Geometry check sheet. Reference: the model listing, model coordinates, mm. A direction names the side the tool comes from. Give positions to 0.01 mm unless a question says otherwise; leave off trailing zeros. Loops run counter-clockwise (first coordinate to the right, second up) from the corner with the lowest first, then second, coordinate; pieces in that order, holes last. Notation, with made-up numbers: (88, 71) - (111, 71) arc R15 ccw to (111, 97) - close; hole circle Ø2 at (29, 3.25). An arc over 180 degrees is marked (long way). Use a Markdown table: item, result. Add a question column.
1. Depth check by flat-ended pin: P1, Ø1.5, axis at y = -0.5, z = -3.5, coming from the +X side; P2, Ø1.5, axis at y = 0, z = -12.5, coming from the -X side; P3, Ø0.9, axis at x = 53.5, y = 0, coming from the -Z side. Enter the tip coordinate at first touch or a pass-through.
2. Cross-section at D-D on x = -9.45. Enter the section's corners in (y, z), and give its area (3 significant figures).
3. Set-up check for faces 1 (the flat face through (15, 0, -24)), 2 (the flat face through (0, 0, 7.9)), 3 (the flat face through (11.6, 0, -6)): record each of +Z, -Z, +X, -X, +Y, -Y from which the full face is reachable in a straight line by a thin tool's end or side.
4. Draft check along X on faces 4 (the flat face through (-43.4, 0, -6)), 5 (the flat face through (45, 0, 9)), 6 (the flat face through (52, 0, -22.6)). Enter one of: pulls with the +X half, pulls with the -X half, needs draft (parallel to the pull), parting line crosses it, or undercut.
5. Cross-section at B-B on y = 0.6. Count the separate pieces of the cut face and the enclosed holes in it, and give its area (3 significant figures).
6. Cross-section at A-A on x = -24.45. Enter the section's corners in (y, z), and give its area (3 significant figures).
7. Material ranges on L1, parallel to X at y = 0.8, z = -23.5; L2, parallel to Z at x = -48, y = -0.3; L3, parallel to Z at x = -14, y = 0.8, recorded low to high.
from build123d import *

# Parameters (mm, degrees)
EXTRUDE_1_DEPTH        = 1.5
SKETCH_2_W             = 94.999999969
SKETCH_2_H             = 7.3
CUT_EXTRUDE_1_DEPTH    = 10
SKETCH_4_W             = 94.999999969
SKETCH_4_H             = 4
CUT_EXTRUDE_3_DEPTH    = 10
SKETCH_5_W             = 30
SKETCH_5_H             = 3
EXTRUDE_2_DEPTH        = 3
EXTRUDE_3_DEPTH        = 3
SKETCH_7_R             = 1
CUT_EXTRUDE_4_DEPTH    = 3
CUT_EXTRUDE_5_DEPTH    = 5
PATTERN_LINEAR_1_COUNT = 19
PATTERN_LINEAR_1_PITCH = 5


with BuildPart() as part:
    # 草图1 → 凸台-拉伸1 (new, symmetric)
    with BuildSketch(Plane(origin=(0, 0, 0), x_dir=(1, 0, 0), z_dir=(0, 1, 0))):
        Polygon((-47.5, 26.6), (-47.5, -15.2), (47.499999969, -15.2), (47.499999969, 26.600010084), align=None)
    extrude(amount=EXTRUDE_1_DEPTH, both=True)

    # 草图2 → 切除-拉伸1 (cut)
    with BuildSketch(Plane(origin=(0, 1.5, 0), x_dir=(1, 0, 0), z_dir=(0, 1, 0))):
        with Locations((-1.5e-08, -11.55)):
            Rectangle(SKETCH_2_W, SKETCH_2_H)
    extrude(amount=-CUT_EXTRUDE_1_DEPTH, mode=Mode.SUBTRACT)

    # 草图4 → 切除-拉伸3 (cut)
    with BuildSketch(Plane(origin=(0, 1.5, 0), x_dir=(1, 0, 0), z_dir=(0, 1, 0))):
        with Locations((-1.5e-08, 24.6)):
            Rectangle(SKETCH_4_W, SKETCH_4_H)
    extrude(amount=-CUT_EXTRUDE_3_DEPTH, mode=Mode.SUBTRACT)


with BuildPart() as cut_extrude_3_kept_piece:
    # of the separate pieces the step leaves, the one the design keeps (cut_extrude_3_pieces_kept)
    add(part.part.solids().sort_by_distance((-47.5, 1.5, -22.6))[0])

    # 草图5 → 凸台-拉伸2 (add)
    with BuildSketch(Plane(origin=(0, 0, -22.6), x_dir=(-1, 0, 0), z_dir=(0, 0, -1))):
        with Locations((30, 0)):
            Rectangle(SKETCH_5_W, SKETCH_5_H)
        with Locations((-30, 0)):
            Rectangle(SKETCH_5_W, SKETCH_5_H)
    extrude_2 = extrude(amount=EXTRUDE_2_DEPTH)

    # 镜向1: 凸台-拉伸2 across plane
    add(extrude_2.mirror(Plane(origin=(0, 0, -7.35), x_dir=(1, 0, 0), z_dir=(0, 0, -1))))

    # 草图8 → 凸台-拉伸3 (add)
    with BuildSketch(Plane(origin=(0, 1.5, 0), x_dir=(1, 0, 0), z_dir=(0, 1, 0))):
        Polygon((-47.5, -7.9), (-47.5, 22.6), (-56.5, 22.6), (-56.5, 16.35), (-53.5, 16.35), (-53.5, -1.65), (-56.5, -1.65), (-56.5, -7.9), align=None)
        Polygon((56.5, -7.9), (56.5, -1.65), (53.5, -1.65), (53.5, 16.35), (56.5, 16.35), (56.5, 22.6), (47.5, 22.6), (47.5, -7.9), align=None)
    extrude(amount=-EXTRUDE_3_DEPTH)

    # 草图7 → 切除-拉伸4 (cut)
    with BuildSketch(Plane(origin=(0, 1.5, 0), x_dir=(1, 0, 0), z_dir=(0, 1, 0))):
        with Locations((-14, 22.6)):
            Circle(SKETCH_7_R)
        with Locations((14, 22.6)):
            Circle(SKETCH_7_R)
        with Locations((46, 22.6)):
            Circle(SKETCH_7_R)
        with Locations((46, -7.9)):
            Circle(SKETCH_7_R)
        with Locations((14, -7.9)):
            Circle(SKETCH_7_R)
        with Locations((-14, -7.9)):
            Circle(SKETCH_7_R)
        with Locations((-46, -7.9)):
            Circle(SKETCH_7_R)
        with Locations((-46, 22.6)):
            Circle(SKETCH_7_R)
        with Locations((-53.5, 15.35)):
            Circle(SKETCH_7_R)
        with Locations((-53.5, -0.65)):
            Circle(SKETCH_7_R)
        with Locations((53.5, -0.65)):
            Circle(SKETCH_7_R)
        with Locations((53.5, 15.35)):
            Circle(SKETCH_7_R)
    extrude(amount=-CUT_EXTRUDE_4_DEPTH, mode=Mode.SUBTRACT)

    # 草图9 → 切除-拉伸5 (cut)
    with BuildSketch(Plane(origin=(0, 1.5, 0), x_dir=(1, 0, 0), z_dir=(0, 1, 0))):
        with BuildLine():
            Line((-45.5, -1.9), (-45.5, 14.1))
            ThreePointArc((-45.5, 14.1), (-44.45, 15.15), (-43.4, 14.1))
            Line((-43.4, 14.1), (-43.4, -1.9))
            ThreePointArc((-43.4, -1.9), (-44.45, -2.95), (-45.5, -1.9))
        make_face()
    cut_extrude_5 = extrude(amount=-CUT_EXTRUDE_5_DEPTH, mode=Mode.SUBTRACT)

    # 阵列(线性)1: 切除-拉伸5 ×19
    with Locations(*[(i * PATTERN_LINEAR_1_PITCH, 0, 0) for i in range(1, PATTERN_LINEAR_1_COUNT)]):
        add(cut_extrude_5, mode=Mode.SUBTRACT)


solid = cut_extrude_3_kept_piece.part
Values found:
| question | item | result |
|---|---|---|
| 1 | P1 | stops at x = 53.5 |
| 1 | P2 | stops at x = -53.5 |
| 1 | P3 | stops at z = -22.6 |
| 2 | outline | (-1.5, -22.6) - (1.5, -22.6) - (1.5, -15.15) - (-1.5, -15.15) - close; (-1.5, 2.95) - (1.5, 2.95) - (1.5, 7.9) - (-1.5, 7.9) - close |
| 2 | area | 37.2 mm2 |
| 3 | face 1 | -Z, +Y, -Y |
| 3 | face 2 | +Z, +Y, -Y |
| 3 | face 3 | +Y, -Y |
| 4 | face 4 | undercut |
| 4 | face 5 | pulls with the +X half |
| 4 | face 6 | needs draft |
| 5 | separate pieces | 1 |
| 5 | enclosed holes | 19 |
| 5 | area | 2,980 mm2 |
| 6 | outline | (-1.5, -25.6) - (1.5, -25.6) - (1.5, -15.15) - (-1.5, -15.15) - close; (-1.5, 2.95) - (1.5, 2.95) - (1.5, 10.9) - (-1.5, 10.9) - close |
| 6 | area | 55.2 mm2 |
| 7 | L1 | x = -45 to -15, 15 to 45 |
| 7 | L2 | z = -22.6 to 7.9 |
| 7 | L3 | z = -21.6 to -15.05, 2.85 to 6.9 |
